The listing builds one solid part. Answer for the finished solid, in the listing's coordinates (mm). Face numbers are marked on the shaded views. Round coordinates to 2 decimals unless told otherwise and drop trailing zeros. Write each loop counter-clockwise with the first axis right and the second up, starting at its lowest first coordinate (ties: lowest second). Pieces come first, ordered by that corner, then holes.
Item 1: Find section A-A on y = 6. Give the vertices of the cut face in (x, z).
Item 2: For a pull along Y with two mould halves and no side action, classify the marked faces 1 and 2 as +Y half, -Y half, draft (parallel to the pull), parting line (faces both ways), or undercut.
Item 3: Find section C-C on y = -5.75. Give the number of separate pieces and of enclosed holes in the cut face, then the cut area to 3 significant figures.
Item 4: Find the intervals of material crossed by probe 1 along X at (y, z) = (7, -3); probe 2 along Z at (x, y) = (-163, 5.25); probe 3 along Z at (x, y) = (-152.25, 3.25), in increasing order.
Item 5: Find section D-D on x = -153.75. Give the vertices of the cut face in (y, z), then the cut area to 4 significant figures.
Item 6: Find section B-B on x = -145. Give the vertices of the cut face in (y, z), then the cut area to 3 significant figures.
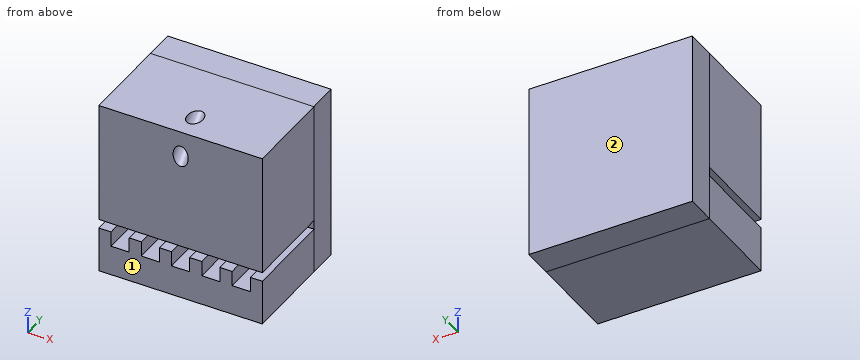
Autodesk Inventor part; units mm, degrees
ref_plane "Work Plane2" through (-258.0475, 7.5, -40.6457) normal (0, 1, 0) x (0, 0, 1)
ref_plane "Work Plane3" through (-258.0475, 7.5, -40.6457) normal (0, 1, 0) x (0, 0, 1)
ref_plane "YZ Plane" through (0, 0, 0) normal (1, 0, 0) x (0, 1, 0)
ref_plane "Work Plane1" through (-17.0854, 0, -12.1778) normal (0, 1, 0) x (0.4190489, 0, 0.9079637)
sketch "Sketch2" plane through (-17.0854, 0, -12.1778) normal (0, 1, 0) x (0.4190489, 0, 0.9079637)
  line L0 (17.3086, 10.8289) -> (-82.3096, -205.0164)
  arc A0 (17.3086, 10.8289) -> (-17.7803, 27.0234) centre (-0.2358, 18.9261) ccw
  line L1 (-117.3985, -188.822) -> (-17.7803, 27.0234)
  arc A1 (-117.3985, -188.822) -> (-82.3096, -205.0164) centre (-99.8541, -196.9192) ccw
  line L2 (-81.4017, -205.4355) -> (18.2166, 10.4099)
  arc A2 (-118.3065, -188.4029) -> (-81.4017, -205.4355) centre (-99.8541, -196.9192) ccw
  line L3 (-18.6883, 27.4424) -> (-118.3065, -188.4029)
  arc A3 (18.2166, 10.4099) -> (-18.6883, 27.4424) centre (-0.2358, 18.9261) ccw
  line L4 (-50.7339, -136.6006) -> (-53.0039, -135.553)
  line L5 (-53.0039, -135.553) -> (-51.7467, -132.8291)
  line L6 (-51.7467, -132.8291) -> (-49.4768, -133.8767)
  line L7 (-48.6387, -132.0608) -> (-50.9086, -131.0132)
  line L8 (-50.9086, -131.0132) -> (-49.6515, -128.2893)
  line L9 (-49.6515, -128.2893) -> (-47.3816, -129.3369)
  line L10 (-46.5435, -127.521) -> (-48.8134, -126.4733)
  line L11 (-48.8134, -126.4733) -> (-47.5562, -123.7494)
  line L12 (-47.5562, -123.7494) -> (-45.2863, -124.7971)
  line L13 (-44.4482, -122.9811) -> (-46.7181, -121.9335)
  line L14 (-46.7181, -121.9335) -> (-45.461, -119.2096)
  line L15 (-45.461, -119.2096) -> (-43.1911, -120.2572)
  line L16 (-42.353, -118.4413) -> (-44.6229, -117.3937)
  line L17 (-44.6229, -117.3937) -> (-43.3657, -114.6698)
  line L18 (-43.3657, -114.6698) -> (-41.0958, -115.7174)
  line L19 (-51.572, -138.4165) -> (-58.3818, -135.2737)
  line L20 (-58.3818, -135.2737) -> (-47.0674, -110.7586)
  line L21 (-47.0674, -110.7586) -> (-40.2577, -113.9015)
  line L22 (-53.8419, -137.3689) -> (-53.0039, -135.553) construction
  line L23 (-51.7467, -132.8291) -> (-50.9086, -131.0132) construction
  line L24 (-43.3657, -114.6698) -> (-42.5276, -112.8539) construction
  line L25 (-40.2577, -113.9015) -> (-38.8958, -114.5301) construction
  line L26 (-38.8958, -114.5301) -> (-50.2101, -139.0451)
  line L27 (-50.2101, -139.0451) -> (-32.0508, -147.4261)
  line L28 (-32.0508, -147.4261) -> (-20.7365, -122.9111)
  line L29 (-20.7365, -122.9111) -> (-38.8958, -114.5301)
  point P0 (-48.6387, -132.0608)
  point P1 (-47.3816, -129.3369)
  point P2 (-45.2863, -124.7971)
  point P3 (-44.4482, -122.9811)
  point P4 (-43.1911, -120.2572)
  point P5 (-42.353, -118.4413)
  point P6 (-41.0958, -115.7174)
  dimension "d9" = 2.5
  dimension "d10" = 3
  dimension "d13" = 5
  dimension "d18" = 5
  dimension "d21" = 1.5
  dimension "d22" = 20
ref_plane "Work Plane2" through (-258.0475, 7.5, -40.6457) normal (0, 1, 0) x (0, 0, 1)
ref_plane "Work Plane3" through (-258.0475, 7.5, -40.6457) normal (0, 1, 0) x (0, 0, 1)
extrude "Extrusion2" add sketch "Sketch2" along normal up to surface (7.5 mm away) contours L0 L18 L17 L16 L15 L14 L13 L12 L11 L10 L9 L8 L7 L6 L5 L4 L19 L20 L21 | L29 L28 L27 L26
sketch "Sketch3" plane through (-164.3738, 7.5, -8.5) normal (0, 1, 0) x (1, 0, 0)
  line L0 (27, -29) -> (27, -9)
  line L1 (0, 0) -> (27, 0)
  line L2 (27, 0) -> (27, -29)
  line L3 (27, -29) -> (0, -29)
  line L4 (0, -29) -> (0, 0)
  point P0 (164.3738, -8.5)
extrude "Extrusion3" add sketch "Sketch3" along normal blind 5
mirror "Mirror1" about plane through (-150.8738, 0, 10.5) normal (0, -1, 0) of "Extrusion2"
ref_plane "Work Plane4" through (-157.6238, -7.5, 20.5) normal (0, -0.7071068, -0.7071068) x (-1, 0, 0)
sketch "Sketch4" plane through (-157.6238, -7.5, 20.5) normal (0, -0.7071068, -0.7071068) x (-1, 0, 0)
  circle A0 centre (-6.75, 3) radius 1.25
  line L0 (-20.25, 28.2843) -> (6.75, 28.2843)
  line L1 (6.75, 28.2843) -> (6.75, 0)
  line L2 (6.75, 0) -> (-20.25, 0)
  line L3 (-20.25, 0) -> (-20.25, 28.2843)
  line L4 (-6.75, 3) -> (-6.75, 0) construction
  point P0 (-157.6238, 19.799)
  dimension "d28" = 2.5
  dimension "d29" = 3
extrude "Extrusion4" cut sketch "Sketch4" against normal through all contours A0
extrude "Extrusion5" cut sketch "Sketch4" along normal through all contours A0
properties part number "Belt Clip"
Check values:
1. outline: (-164.37, -8.5) - (-137.37, -8.5) - (-137.37, -1) - (-139.37, -1) - (-139.37, -3.5) - (-142.37, -3.5) - (-142.37, -1) - (-144.37, -1) - (-144.37, -3.5) - (-147.37, -3.5) - (-147.37, -1) - (-149.37, -1) - (-149.37, -3.5) - (-152.37, -3.5) - (-152.37, -1) - (-154.37, -1) - (-154.37, -3.5) - (-157.37, -3.5) - (-157.37, -1) - (-159.37, -1) - (-159.37, -3.5) - (-162.37, -3.5) - (-162.37, -1) - (-164.37, -1) - close; (-164.37, 0.5) - (-137.37, 0.5) - (-137.37, 20.5) - (-164.37, 20.5) - close
2. face 1: -Y half
2. face 2: +Y half
3. separate pieces: 2
3. enclosed holes: 1
3. area: 698 mm2
4. probe 1: x = -164.37 to -162.37, -159.37 to -157.37, -154.37 to -152.37, -149.37 to -147.37, -144.37 to -142.37, -139.37 to -137.37
4. probe 2: z = -8.5 to -1, 0.5 to 20.5
4. probe 3: z = -8.5 to -3.5, 0.5 to 20.5
5. outline: (-7.5, -8.5) - (12.5, -8.5) - (12.5, 20.5) - (-7.5, 20.5) - (-7.5, 0.5) - (7.5, 0.5) - (7.5, -1) - (-7.5, -1) - close
5. area: 557.5 mm2
6. outline: (-7.5, -8.5) - (12.5, -8.5) - (12.5, 20.5) - (-7.5, 20.5) - (-7.5, 0.5) - (7.5, 0.5) - (7.5, -3.5) - (-7.5, -3.5) - close
6. area: 520 mm2
